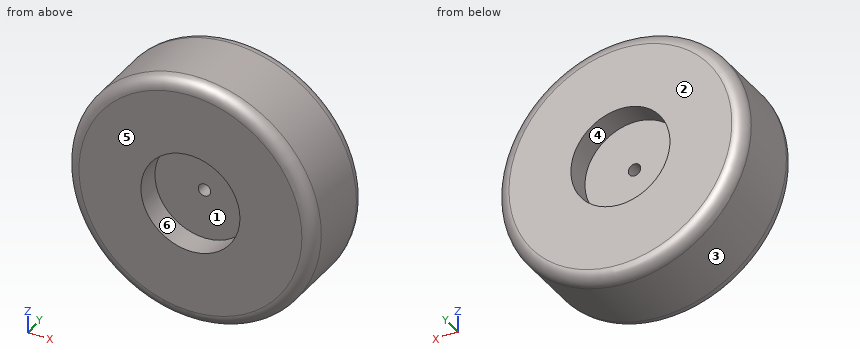
from build123d import *

# Parameters (mm, degrees)
F0_R      = 254
F1_DEPTH  = 88.9
F2_R      = 101.6
F3_DEPTH  = 63.5
F8_R      = 101.6
F9_DEPTH  = 177.8
F10_R     = 101.6
F11_DEPTH = 38.1
F12_R     = 25.4
F13_R     = 12.7
F14_DEPTH = 177.8


# Not quite as in the source:
# - a feature of the source that left no trace in its solid (it failed there, or was rolled back) is left out
# - a pattern or mirror of a feature is missing from the dataset's text; its kind, count and spacing are read off the source's solid


with BuildPart() as f1:
    # F0 (on Front) → F1 (new body, symmetric)
    with BuildSketch(Plane.XZ):
        Circle(F0_R)
    extrude(amount=F1_DEPTH, both=True)

    # F2 (on face) → F3 (cut, symmetric)
    with BuildSketch(Plane.XZ.offset(88.9)):
        Circle(F2_R)
    f3 = extrude(amount=F3_DEPTH, both=True, mode=Mode.SUBTRACT)

    # F3_copies: F3 across plane
    add(f3.mirror(Plane.ZX), mode=Mode.SUBTRACT)

    # F8 (on face) → F9 (cut, symmetric)
    with BuildSketch(Plane.XZ.offset(152.4)):
        Circle(F8_R)
    extrude(amount=F9_DEPTH, both=True, mode=Mode.SUBTRACT)

    # F10 (on Front) → F11 (join, symmetric)
    with BuildSketch(Plane.XZ):
        Circle(F10_R)
    extrude(amount=F11_DEPTH, both=True)

    # F12
    f12_edges = [f1.edges().sort_by_distance(p)[0] for p in [
        (-254, 88.9, 0),
        (-254, -88.9, 0),
    ]]
    fillet(f12_edges, radius=F12_R)

    # F13 (on face) → F14 (cut, symmetric)
    with BuildSketch(Plane(origin=(0, 38.1, 0), x_dir=(-1, 0, 0), z_dir=(0, 1, 0))):
        Circle(F13_R)
    extrude(amount=F14_DEPTH, both=True, mode=Mode.SUBTRACT)


solid = f1.part
Geometry check sheet. Reference: the model listing, model coordinates, mm. Face numbers are marked on the shaded views. A direction names the side the tool comes from. Round coordinates to 2 decimals unless told otherwise and drop trailing zeros. Loops run counter-clockwise (first coordinate to the right, second up) from the corner with the lowest first, then second, coordinate; pieces in that order, holes last. Notation, with made-up numbers: (-28, 87.25) - (-16, 87.25) arc R30 cw to (-16, 122.25) - close; hole circle Ø1 at (64.5, -30). An arc over 180 degrees is marked (long way). One line per question, with ' | ' between items. Start each with the question number.
1. Cross-section at C-C on y = 27.5. Record the cut outline in (x, z).
2. Tool access check on the marked faces 4, 5 and 6. Record the directions out of +Z, -Z, +X, -X, +Y, -Y that give a thin tool (end or side, any length) a straight path to the whole face; none if there is none.
3. Cross-section at A-A on z = 0. Record the cut outline in (x, y).
4. Draft check along X on the marked faces 1, 2 and 3. Enter one of: released by +X, released by -X, zero draft, split by the parting line, or undercut.
5. Cross-section at B-B on x = 0. Record the cut outline in (y, z).
6. Scan lines: line 1 (Z direction, x = 0, y = 17); line 2 (X direction, y = 43, z = 24.5); line 3 (X direction, y = -20, z = 3). Record each from-to range of solid material in increasing order. Write a range as [from, to].
7. Depth check by flat-ended pin: pin 1 (3 mm diameter, centred on y = 6, z = 174, fed in from +X); pin 2 (5 mm diameter, centred on y = -64, z = -152, fed in from -X); pin 3 (1.5 mm diameter, centred on x = -134.5, y = 16, fed in from +Z). Enter the tip coordinate at first touch or a pass-through.
8. Cross-section at D-D on y = -56. Record the cut outline in (x, z), then the cut area to 3 significant figures.
Taken from the geometry:
1) outline: circle Ø508 at (0, 0); hole circle Ø25.4 at (0, 0)
2) face 4: +Y | face 5: +Z, -Z, +X, -X, -Y | face 6: -Y
3) outline: (-254, -63.5) arc R25.4 ccw to (-228.6, -88.9) - (-101.6, -88.9) - (-101.6, -38.1) - (-12.7, -38.1) - (-12.7, 38.1) - (-101.6, 38.1) - (-101.6, 88.9) - (-228.6, 88.9) arc R25.4 ccw to (-254, 63.5) - close; (12.7, -38.1) - (101.6, -38.1) - (101.6, -88.9) - (228.6, -88.9) arc R25.4 ccw to (254, -63.5) - (254, 63.5) arc R25.4 ccw to (228.6, 88.9) - (101.6, 88.9) - (101.6, 38.1) - (12.7, 38.1) - close
4) face 1: undercut | face 2: zero draft | face 3: split by the parting line
5) outline: (-88.9, -228.6) arc R25.4 ccw to (-63.5, -254) - (63.5, -254) arc R25.4 ccw to (88.9, -228.6) - (88.9, -101.6) - (38.1, -101.6) - (38.1, -12.7) - (-38.1, -12.7) - (-38.1, -101.6) - (-88.9, -101.6) - close; (-88.9, 101.6) - (-38.1, 101.6) - (-38.1, 12.7) - (38.1, 12.7) - (38.1, 101.6) - (88.9, 101.6) - (88.9, 228.6) arc R25.4 ccw to (63.5, 254) - (-63.5, 254) arc R25.4 ccw to (-88.9, 228.6) - close
6) line 1: [-254, -12.7], [12.7, 254] | line 2: [-252.82, -98.6], [98.6, 252.82] | line 3: [-253.98, -12.34], [12.34, 253.98]
7) pin 1: x = 186.44 | pin 2: x = -205.34 | pin 3: z = 215.93
8) outline: circle Ø508 at (0, 0); hole circle Ø203.2 at (0, 0) | area: 170,000 mm²
